The drawing under review shows one solid part. Ordinate dimensions are in mm from its lowest x, y, z. Coordinates: 2 decimals unless noted, no trailing zeros. Order: outer loops, then holes, each group sorted by start corner. A loop starts at its lowest first (then second) coordinate and runs counter-clockwise, first axis right, second up.
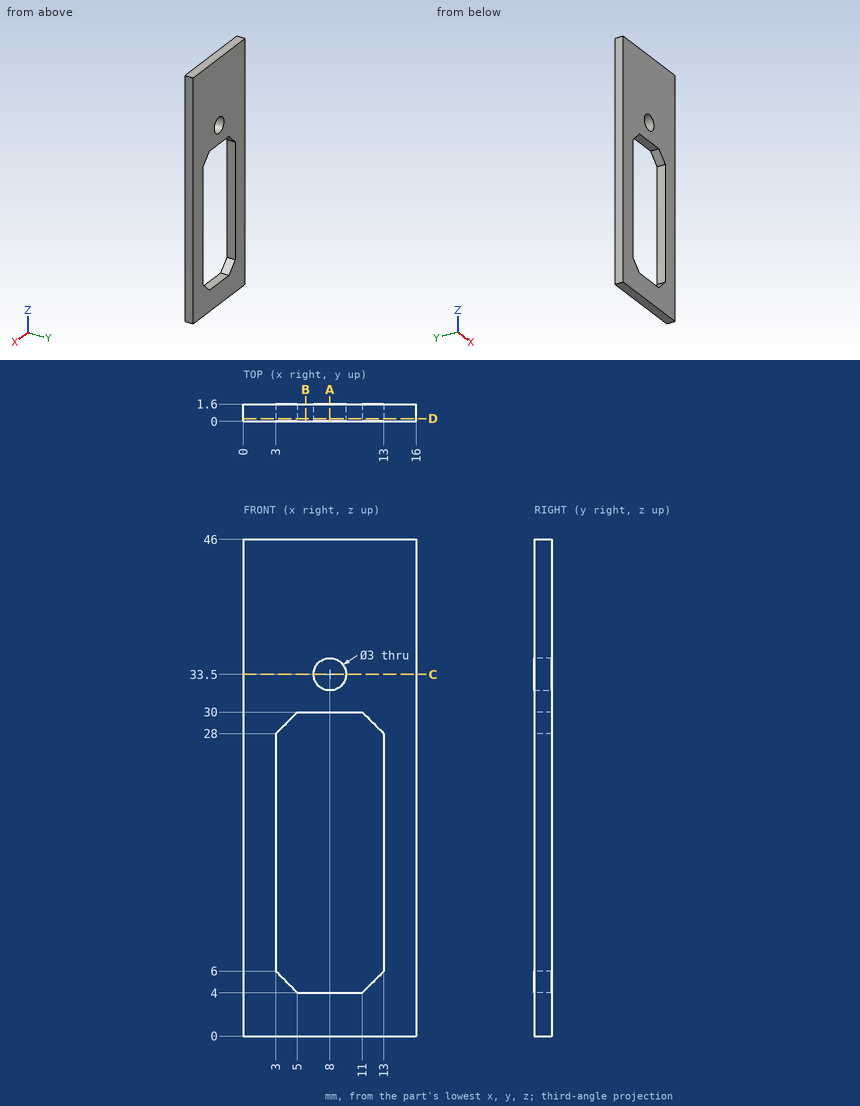
(1) Wall thickness on line 1 (X direction, y = 0.9, z = 17); line 2 (X direction, y = 1.05, z = 33.5); line 3 (Z direction, x = 9.25, y = 1.4): over which ranges is each line inside the solid? List them lowest first.
(2) Consider section A-A (x = 8). Give the boundary of the cut face in (y, z).
(3) Consider section D-D (y = 0.25). Give the boundary of the cut face in (x, z).
(4) Consider section C-C (z = 33.5). Give the boundary of the cut face in (x, y).
(5) Consider section B-B (x = 5.75). Give the boundary of the cut face in (y, z).
Findings:
1. line 1: x = 0 to 3, 13 to 16
1. line 2: x = 0 to 6.5, 9.5 to 16
1. line 3: z = 0 to 4, 30 to 32.67, 34.33 to 46
2. outline: (0, 0) - (1.6, 0) - (1.6, 4) - (0, 4) - close; (0, 30) - (1.6, 30) - (1.6, 32) - (0, 32) - close; (0, 35) - (1.6, 35) - (1.6, 46) - (0, 46) - close
3. outline: (0, 0) - (16, 0) - (16, 46) - (0, 46) - close; hole (3, 6) - (5, 4) - (11, 4) - (13, 6) - (13, 28) - (11, 30) - (5, 30) - (3, 28) - close; hole circle Ø3 at (8, 33.5)
4. outline: (0, 0) - (6.5, 0) - (6.5, 1.6) - (0, 1.6) - close; (9.5, 0) - (16, 0) - (16, 1.6) - (9.5, 1.6) - close
5. outline: (0, 0) - (1.6, 0) - (1.6, 4) - (0, 4) - close; (0, 30) - (1.6, 30) - (1.6, 46) - (0, 46) - close
